from build123d import *

# Parameters (mm, degrees)
SKETCH1_W               = 75
SKETCH1_H               = 12.7
LOADCELL_DEPTH          = 6.35
SKETCH2_R               = 2
CUT_EXTRUDE1_DEPTH      = 7.35
CUT_EXTRUDE1_DEPTH_BACK = 7.35


with BuildPart() as part:
    # Sketch1 → LoadCell (new body, symmetric)
    with BuildSketch(Plane.XY):
        Rectangle(SKETCH1_W, SKETCH1_H)
        with BuildLine():
            ThreePointArc((0, 3.681901683), (-8.58, 0), (0, -3.681901683))
            ThreePointArc((0, -3.681901683), (8.58, 0), (0, 3.681901683))
        make_face(mode=Mode.SUBTRACT)
    extrude(amount=LOADCELL_DEPTH, both=True)

    # Sketch2 → Cut-Extrude1 (cut, two sides)
    with BuildSketch(Plane(origin=(0, 0, 0), x_dir=(1, 0, 0), z_dir=(0, 1, 0))) as cut_extrude1_sk:
        with Locations((-31.999999942, 0)):
            Circle(SKETCH2_R)
        with Locations((-21.999999942, 0)):
            Circle(SKETCH2_R)
        with Locations((31.999999942, 0)):
            Circle(SKETCH2_R)
        with Locations((21.999999942, 0)):
            Circle(SKETCH2_R)
    extrude(amount=CUT_EXTRUDE1_DEPTH, mode=Mode.SUBTRACT)
    extrude(cut_extrude1_sk.sketch, amount=-CUT_EXTRUDE1_DEPTH_BACK, mode=Mode.SUBTRACT)


solid = part.part
Work out the finished part from the listing and answer in its coordinate system (mm). Give positions to 0.01 mm unless a question says otherwise; leave off trailing zeros. Order: outer loops, then holes, each group sorted by start corner. A loop starts at its lowest first (then second) coordinate and runs counter-clockwise, first axis right, second up. Notation, with made-up numbers: (47, 84.5) -> (66, 84.5) arc R21 ccw to (66, 116.5) -> close; hole circle Ø2 at (-14.75, -23). An arc over 180 degrees is marked (long way). One line per item, written item: value.
Item 1: Find section C-C, the plane z = 0. Give the vertices of the cut face in (x, y).
Answer sheet:
outline: (-37.5, -6.35) -> (-34, -6.35) -> (-34, 6.35) -> (-37.5, 6.35) -> close; (-30, -6.35) -> (-24, -6.35) -> (-24, 6.35) -> (-30, 6.35) -> close; (-20, -6.35) -> (20, -6.35) -> (20, 6.35) -> (-20, 6.35) -> close; (24, -6.35) -> (30, -6.35) -> (30, 6.35) -> (24, 6.35) -> close; (34, -6.35) -> (37.5, -6.35) -> (37.5, 6.35) -> (34, 6.35) -> close; hole (0, -3.68) arc R5.08 ccw (long way) to (0, 3.68) arc R5.08 ccw (long way) to start
Item 2: Find section B-B, the plane x = -22. Give the vertices of the cut face in (y, z), plus the area to 3 significant figures.
Answer sheet:
outline: (-6.35, -6.35) -> (6.35, -6.35) -> (6.35, -2) -> (-6.35, -2) -> close; (-6.35, 2) -> (6.35, 2) -> (6.35, 6.35) -> (-6.35, 6.35) -> close
area: 110 mm²
Item 3: Find section A-A, the plane y = 1. Give the vertices of the cut face in (x, z).
Answer sheet:
outline: (-37.5, -6.35) -> (-8.48, -6.35) -> (-8.48, 6.35) -> (-37.5, 6.35) -> close; (8.48, -6.35) -> (37.5, -6.35) -> (37.5, 6.35) -> (8.48, 6.35) -> close; hole circle Ø4 at (-32, 0); hole circle Ø4 at (-22, 0); hole circle Ø4 at (22, 0); hole circle Ø4 at (32, 0)
Item 4: Straight lines are drawn through the part: probe 1 along X at (y, z) = (0.25, 1.5); probe 2 along X at (y, z) = (-1.25, 0); probe 3 along Z at (x, y) = (22, -1.25). For each, find the intervals that lie inside material, in ascending order.
Answer sheet:
probe 1: -37.5 to -33.32, -30.68 to -23.32, -20.68 to -8.57, 8.57 to 20.68, 23.32 to 30.68, 33.32 to 37.5
probe 2: -37.5 to -34, -30 to -24, -20 to -8.42, 8.42 to 20, 24 to 30, 34 to 37.5
probe 3: -6.35 to -2, 2 to 6.35
Item 5: Determine the mould class of faces 1 (the cylindrical face through (30, 0, 0)), 2 (the flat face through (-0.5, 4.3, 6.35)), 3 (the flat face through (-1, 6.35, 0)) for opening direction Z: released by +Z, released by -Z, zero draft, split by the parting line, or undercut.
Answer sheet:
face 1: undercut
face 2: released by +Z
face 3: zero draft
Item 6: Find section D-D, the plane x = 3.5. Give the vertices of the cut face in (y, z).
Answer sheet:
outline: (-6.35, -6.35) -> (-5.08, -6.35) -> (-5.08, 6.35) -> (-6.35, 6.35) -> close; (5.08, -6.35) -> (6.35, -6.35) -> (6.35, 6.35) -> (5.08, 6.35) -> close
